```python
from build123d import *

# Parameters (mm, degrees)
SKETCH1_W           = 240
SKETCH1_H           = 240
SKETCH1_R           = 20
SKETCH1_R_2         = 5.5
BOSS_EXTRUDE1_DEPTH = 15
SKETCH2_R           = 70
SKETCH2_R_2         = 20
BOSS_EXTRUDE2_DEPTH = 75
SKETCH3_R           = 80
SKETCH3_R_2         = 40
SKETCH3_R_3         = 3
BOSS_EXTRUDE3_DEPTH = 25


with BuildPart() as part:
    # Sketch1 → Boss-Extrude1 (new body)
    with BuildSketch(Plane.XY):
        Rectangle(SKETCH1_W, SKETCH1_H)
        Circle(SKETCH1_R, mode=Mode.SUBTRACT)
        with Locations((-95, -95)):
            Circle(SKETCH1_R_2, mode=Mode.SUBTRACT)
        with Locations((-95, 95)):
            Circle(SKETCH1_R_2, mode=Mode.SUBTRACT)
        with Locations((95, -95)):
            Circle(SKETCH1_R_2, mode=Mode.SUBTRACT)
        with Locations((95, 95)):
            Circle(SKETCH1_R_2, mode=Mode.SUBTRACT)
    extrude(amount=BOSS_EXTRUDE1_DEPTH)

    # Sketch2 → Boss-Extrude2 (add)
    with BuildSketch(Plane.XY):
        with Locations(Location((0, 0, 0), (0, 0, 180))):
            Circle(SKETCH2_R)
        Circle(SKETCH2_R_2, mode=Mode.SUBTRACT)
    extrude(amount=BOSS_EXTRUDE2_DEPTH)

    # Sketch3 → Boss-Extrude3 (add)
    with BuildSketch(Plane.XY):
        with Locations(Location((0, 0, 0), (0, 0, 180))):
            Circle(SKETCH3_R)
        Circle(SKETCH3_R_2, mode=Mode.SUBTRACT)
        with Locations((65, 0)):
            Circle(SKETCH3_R_3, mode=Mode.SUBTRACT)
        with Locations((45.961940777, 45.961940777)):
            Circle(SKETCH3_R_3, mode=Mode.SUBTRACT)
        with Locations((0, 65)):
            Circle(SKETCH3_R_3, mode=Mode.SUBTRACT)
        with Locations((-45.961940777, 45.961940777)):
            Circle(SKETCH3_R_3, mode=Mode.SUBTRACT)
        with Locations((-65, 0)):
            Circle(SKETCH3_R_3, mode=Mode.SUBTRACT)
        with Locations((-45.961940777, -45.961940777)):
            Circle(SKETCH3_R_3, mode=Mode.SUBTRACT)
        with Locations((0, -65)):
            Circle(SKETCH3_R_3, mode=Mode.SUBTRACT)
        with Locations((45.961940777, -45.961940777)):
            Circle(SKETCH3_R_3, mode=Mode.SUBTRACT)
    extrude(amount=BOSS_EXTRUDE3_DEPTH)


solid = part.part
```
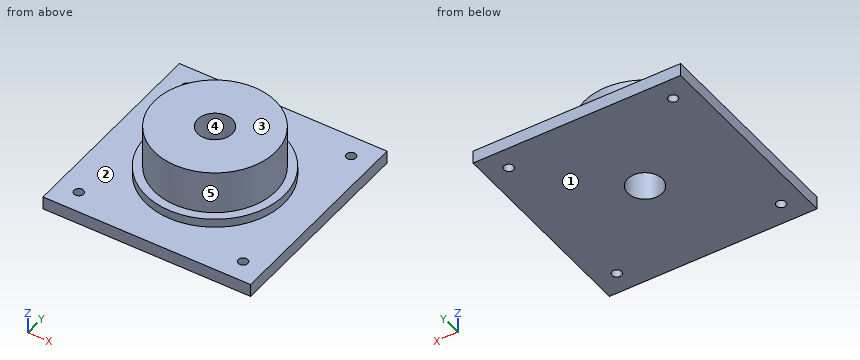
For this review, take the finished solid that the model builds, in its own axes (mm). Face numbers are marked on the shaded views. A direction names the side the tool comes from. Coordinates: 2 decimals unless noted, no trailing zeros. Order: outer loops, then holes, each group sorted by start corner. A loop starts at its lowest first (then second) coordinate and runs counter-clockwise, first axis right, second up. Notation, with made-up numbers: (-19, 0) -> (36, 0) arc R21 cw to (36, 25) -> close; hole circle Ø8 at (-27.5, -21.5). An arc over 180 degrees is marked (long way). Use CSV: the item, a comma, the result in double quotes. Start each with the question number.
Item 1: Wall thickness on probe 1 along Y at (x, z) = (-95, 7); probe 2 along Z at (x, y) = (84, 27); probe 3 along Y at (x, z) = (0, 16.5): over which ranges is each line inside the solid? List them lowest first.
Item 2: We need section A-A, the plane y = 0. Give the boundary of the cut face in (x, z).
Item 3: Draft analysis for pull direction Y (two halves, no side actions). For the marked faces 3, 4 and 5, state which applies: pulls with the +Y half, pulls with the -Y half, needs draft (parallel to the pull), parting line crosses it, or undercut.
Item 4: We need section B-B, the plane y = -95. Give the boundary of the cut face in (x, z), then the cut area to 3 significant figures.
Item 5: Insertion check: pin 1 (6 mm diameter, centred on x = -65, z = 43, fed in from +Y); pin 2 (1.5 mm diameter, centred on y = 48, z = 60.5, fed in from +X); pin 3 (2 mm diameter, centred on x = 11.5, z = 31.5, fed in from +Y). Each pin has a flat end and moves straight along its axis. Give the tip position at first contact, or say it passes through.
Item 6: For the marked faces 1 and 2, list the 3-axis set-ups (+Z, -Z, +X, -X, +Y, -Y) from which the entire face can be reached by the end or side of a thin tool; tool diameter is ignored.
Item 7: We need section D-D, the plane z = 60. Give the boundary of the cut face in (x, y), then the cut area to 3 significant figures.
Derived:
1,probe 1,"y = -120 to -100.5, -89.5 to 89.5, 100.5 to 120"
1,probe 2,"z = 0 to 15"
1,probe 3,"y = -80 to -20, 20 to 80"
2,outline,"(-120, 0) -> (-20, 0) -> (-20, 75) -> (-70, 75) -> (-70, 25) -> (-80, 25) -> (-80, 15) -> (-120, 15) -> close; (20, 0) -> (120, 0) -> (120, 15) -> (80, 15) -> (80, 25) -> (70, 25) -> (70, 75) -> (20, 75) -> close"
3,face 3,"needs draft"
3,face 4,"undercut"
3,face 5,"parting line crosses it"
4,outline,"(-120, 0) -> (-100.5, 0) -> (-100.5, 15) -> (-120, 15) -> close; (-89.5, 0) -> (89.5, 0) -> (89.5, 15) -> (-89.5, 15) -> close; (100.5, 0) -> (120, 0) -> (120, 15) -> (100.5, 15) -> close"
4,area,"3,270 mm^2"
5,pin 1,"stops at y = 32.5"
5,pin 2,"stops at x = 51.65"
5,pin 3,"stops at y = 69.21"
6,face 1,"-Z, +X, -X, +Y, -Y"
6,face 2,"+Z"
7,outline,"circle Ø140 at (0, 0); hole circle Ø40 at (0, 0)"
7,area,"14,100 mm^2"
